from build123d import *

# Parameters (mm, degrees)
F0_W      = 67
F0_H      = 138
F1_DEPTH  = 10
F2_T      = -2.54
F3_R      = 5.08
F4_R      = 5.08
F5_R      = 5.08
F6_R      = 5.08
F7_W      = 26.614272967
F7_H      = 10.362688452
F8_DEPTH  = 25.4
F9_W      = 22.4436074495
F9_H      = 4.9550822005
F10_DEPTH = 12.7
F11_W     = 24.2274198681
F11_H     = 4.6703449916
F12_DEPTH = 25.4
F13_W     = 20.1118066907
F13_H     = 4.9550810363
F14_DEPTH = 25.4


with BuildPart() as f1:
    # F0 (on Top) → F1 (new body)
    with BuildSketch(Plane.XY):
        with Locations((-11.3872148991, -5.1804912686)):
            Rectangle(F0_W, F0_H)
    extrude(amount=F1_DEPTH)

    # F2
    f2_openings = [f1.faces().sort_by_distance(p)[0] for p in [
        (-11.387215, -5.180491, 10),
    ]]
    offset(amount=F2_T, openings=f2_openings)

    # F3
    f3_edges = [f1.edges().sort_by_distance(p)[0] for p in [
        (-44.887215, 63.819509, 5),
    ]]
    fillet(f3_edges, radius=F3_R)

    # F4
    f4_edges = [f1.edges().sort_by_distance(p)[0] for p in [
        (22.112785, 63.819509, 5),
    ]]
    fillet(f4_edges, radius=F4_R)

    # F5
    f5_edges = [f1.edges().sort_by_distance(p)[0] for p in [
        (22.112785, -74.180491, 5),
    ]]
    fillet(f5_edges, radius=F5_R)

    # F6
    f6_edges = [f1.edges().sort_by_distance(p)[0] for p in [
        (-44.887215, -74.180491, 5),
    ]]
    fillet(f6_edges, radius=F6_R)

    # F7 (on face) → F8 (cut)
    with BuildSketch(Plane(origin=(0, 0, 0), x_dir=(1, 0, 0), z_dir=(0, 0, -1))):
        with Locations((1.5710769221, -56.3431996852)):
            Rectangle(F7_W, F7_H)
        with BuildLine():
            Line((14.8782134056, -51.1618554592), (14.8782134056, -61.5245439112))
            ThreePointArc((14.8782134056, -61.5245439112), (20.0595576316, -56.3431996852), (14.8782134056, -51.1618554592))
        make_face()
        with BuildLine():
            ThreePointArc((-11.7360595614, -51.1618554592), (-16.9174037874, -56.3431996852), (-11.7360595614, -61.5245439112))
            Line((-11.7360595614, -61.5245439112), (-11.7360595614, -51.1618554592))
        make_face()
    extrude(amount=-F8_DEPTH, mode=Mode.SUBTRACT)

    # F9 (on face) → F10 (cut, symmetric)
    with BuildSketch(Plane.XZ.offset(74.1804912686)):
        with Locations((-11.2218037248, 4.9550822005)):
            Rectangle(F9_W, F9_H)
    extrude(amount=F10_DEPTH, both=True, mode=Mode.SUBTRACT)

    # F11 (on face) → F12 (cut)
    with BuildSketch(Plane(origin=(-44.8872148991, 0, 0), x_dir=(0, -1, 0), z_dir=(-1, 0, 0))):
        with Locations((-42.2179875895, 5.0382829504)):
            Rectangle(F11_W, F11_H)
    extrude(amount=-F12_DEPTH, mode=Mode.SUBTRACT)

    # F13 (on face) → F14 (cut)
    with BuildSketch(Plane.YZ.offset(22.1127851009)):
        with Locations((44.3042628467, 5.1008212613)):
            Rectangle(F13_W, F13_H)
    extrude(amount=-F14_DEPTH, mode=Mode.SUBTRACT)


solid = f1.part
Here's how the part is built. I have some questions about the finished solid (model axes, mm). A direction names the side the tool comes from. Round coordinates to 2 decimals unless told otherwise and drop trailing zeros. Write each loop counter-clockwise with the first axis right and the second up, starting at its lowest first coordinate (ties: lowest second). Pieces come first, ordered by that corner, then holes. Notation, with made-up numbers: (26, 70) -> (83, 70) arc R35 cw to (83, 105) -> close; hole circle Ø9 at (-1.5, 34.25). An arc over 180 degrees is marked (long way). One line per item, written item: value.
1) Suppose I cut it at B-B on x = 6.5. List the corners of the cut face in (y, z) for me.
Filled sheet:
outline: (-74.18, 0) -> (51.16, 0) -> (51.16, 2.54) -> (-71.64, 2.54) -> (-71.64, 10) -> (-74.18, 10) -> close; (61.52, 0) -> (63.82, 0) -> (63.82, 10) -> (61.52, 10) -> close
2) We'd pull the mould along Z, two halves only. Please class faces 4 (the face through (19, 61, 2.54)), 5 (the face through (21, 34.248, 5)), 6 (the face through (22.113, -6, 5)), 7 (the face through (-44, 30.104, 5)): released by +Z, released by -Z, zero draft, split by the parting line, or undercut.
Filled sheet:
face 4: released by +Z
face 5: undercut
face 6: zero draft
face 7: undercut
3) Suppose I cut it at C-C on z = 5.25. Give the number of separate pieces and of enclosed holes in the cut face, plus the area to 3 significant figures.
Filled sheet:
separate pieces: 3
enclosed holes: 0
area: 815 mm2
4) Suppose I cut it at A-A on y = 47. List the corners of the cut face in (x, z) for me.
Filled sheet:
outline: (-44.89, 0) -> (22.11, 0) -> (22.11, 2.62) -> (19.57, 2.62) -> (19.57, 2.54) -> (-42.35, 2.54) -> (-42.35, 2.7) -> (-44.89, 2.7) -> close; (-44.89, 7.37) -> (-42.35, 7.37) -> (-42.35, 10) -> (-44.89, 10) -> close; (19.57, 7.58) -> (22.11, 7.58) -> (22.11, 10) -> (19.57, 10) -> close
5) If I drill on line 1 (X direction, y = -33, z = 9); line 2 (Y direction, x = 14, z = 7.25); line 3 (Y direction, x = -32, z = 4), over which ranges is the centre line in solid material (lowest first)? Write a range as [from, to].
Filled sheet:
line 1: x = [-44.89, -42.35], [19.57, 22.11]
line 2: y = [-74.18, -71.64], [61.52, 63.82]
line 3: y = [-74.18, -71.64], [61.28, 63.82]
6) Suppose I cut it at D-D on x = -5.5. List the corners of the cut face in (y, z) for me, plus the area to 3 significant figures.
Filled sheet:
outline: (-74.18, 0) -> (51.16, 0) -> (51.16, 2.54) -> (-61.48, 2.54) -> (-61.48, 2.48) -> (-74.18, 2.48) -> close; (-74.18, 7.43) -> (-71.64, 7.43) -> (-71.64, 10) -> (-74.18, 10) -> close; (61.52, 0) -> (63.82, 0) -> (63.82, 10) -> (61.52, 10) -> close
area: 347 mm2
7) For faces 1 (the face through (19.707, 58.222, 3.819)), 2 (the face through (-44, 54.332, 5)), 3 (the face through (-42.347, -21, 6)), which set-ups out of +Z, -Z, +X, -X, +Y, -Y let a thin tool reach every point of the face, with its end or its side?
Filled sheet:
face 1: +Z, -Z
face 2: +X, -X
face 3: +Z
8) I'm going to push flat-ended pins straight in: pin 1 Ø5 at (x, y) = (-16, -55) entering from +Z; pin 2 Ø0.8 at (x, z) = (21, 6) entering from +Y; pin 3 Ø0.8 at (x, z) = (-44, 4.5) entering from +Y. Where does each tip first touch, or does it pass through?
Filled sheet:
pin 1: stops at z = 2.54
pin 2: stops at y = 62.36
pin 3: stops at y = 62.12
